```python
from build123d import *

# Parameters (mm, degrees)
F0_R     = 35.27027
F0_R_2   = 25.372409
F1_DEPTH = 50.8
F2_W     = 48.85688
F2_H     = 53.797463
F3_DEPTH = 25.4
F5_DEPTH = 5.08


with BuildPart() as f1:
    # F0 (on Top) → F1 (new body)
    with BuildSketch(Plane.XY):
        with Locations((0, 35.27027)):
            Circle(F0_R)
        with Locations((0, 35.27027)):
            Circle(F0_R_2, mode=Mode.SUBTRACT)
    extrude(amount=F1_DEPTH)

    # F2 (on Top) → F3 (join)
    with BuildSketch(Plane.XY):
        with Locations((0, -17.154805)):
            Rectangle(F2_W, F2_H)
    extrude(amount=F3_DEPTH)

    # F4 (on Right) → F5 (join, symmetric)
    with BuildSketch(Plane.YZ):
        Polygon((-27.996639, 25.663584), (4.117153, 25.389109), (4.117153, 41.857719), align=None)
    extrude(amount=F5_DEPTH, both=True)


solid = f1.part
```
Geometry check sheet. Reference: the model listing, model coordinates, mm. A direction names the side the tool comes from. Round coordinates to 2 decimals unless told otherwise and drop trailing zeros. Loops run counter-clockwise (first coordinate to the right, second up) from the corner with the lowest first, then second, coordinate; pieces in that order, holes last. Notation, with made-up numbers: (45, 52.25) -> (95, 52.25) arc R14 cw to (95, 76.25) -> close; hole circle Ø5 at (61, 11). An arc over 180 degrees is marked (long way). Use a Markdown table: item, result.
(1) Go/stop test with flat-tipped pins: P1, Ø12.5, axis at y = -28, z = 12.5, coming from the -X side; P2, Ø24.5, axis at x = -0.5, y = -17.5, coming from the +Z side; P3, Ø2, axis at y = 13, z = 22, coming from the +X side. Record where each tip stops, or that it passes through.
Calculated:
| item | result |
|---|---|
| P1 | x = -24.43 |
| P2 | z = 37.13 |
| P3 | x = 28.13 |
(2) Scan lines: probe 1 along Y at (x, z) = (0, 15); probe 2 along X at (y, z) = (-1, 12); probe 3 along Z at (x, y) = (-16, -33.5). Record each from-to range of solid material in increasing order.
Calculated:
| item | result |
|---|---|
| probe 1 | -44.05 to 9.9, 60.64 to 70.54 |
| probe 2 | -24.43 to 24.43 |
| probe 3 | 0 to 25.4 |
(3) Sectioned sample at A-A (y = 31). Enter the section's corners in (x, z), then the cut area to 3 significant figures.
Calculated:
| item | result |
|---|---|
| outline | (-35.01, 0) -> (-25.01, 0) -> (-25.01, 50.8) -> (-35.01, 50.8) -> close; (25.01, 0) -> (35.01, 0) -> (35.01, 50.8) -> (25.01, 50.8) -> close |
| area | 1,020 mm² |
(4) Sectioned sample at D-D (x = 22.5). Enter the section's corners in (y, z), then the cut area to 3 significant figures.
Calculated:
| item | result |
|---|---|
| outline | (-44.05, 0) -> (23.54, 0) -> (23.54, 50.8) -> (8.11, 50.8) -> (8.11, 25.4) -> (-44.05, 25.4) -> close; (47, 0) -> (62.43, 0) -> (62.43, 50.8) -> (47, 50.8) -> close |
| area | 2,890 mm² |
(5) Mould release check, pull along X, two halves, no side actions. Record for faces 6 (the flat face through (-5.08, -11, 30)), 7 (the flat face through (-24, 44, 50.8)), 8 (the cylindrical face through (-3.303, 60.427, 25.044)): released by +X, released by -X, zero draft, split by the parting line, or undercut.
Calculated:
| item | result |
|---|---|
| face 6 | released by -X |
| face 7 | zero draft |
| face 8 | undercut |
(6) Sectioned sample at C-C (z = 38.5). Enter the section's corners in (x, y).
Calculated:
| item | result |
|---|---|
| outline | (-5.08, -2.54) -> (5.08, -2.54) -> (5.08, 0.37) arc R35.27 ccw (long way) to (-5.08, 0.37) -> close; hole circle Ø50.74 at (0, 35.27) |
(7) Set-up check for faces 1 (the flat face through (0, 1, 0)), 2 (the flat face through (5.08, -11, 30)), 3 (the flat face through (0, -44.054, 13)), 4 (the flat face through (24.428, -18, 13)), 5 (the flat face through (-24.428, -18, 13)): record each of +Z, -Z, +X, -X, +Y, -Y from which the full face is reachable in a straight line by a thin tool's end or side.
Calculated:
| item | result |
|---|---|
| face 1 | -Z, +X, -X, +Y, -Y |
| face 2 | +Z, +X, -Y |
| face 3 | +Z, -Z, +X, -X, -Y |
| face 4 | +Z, -Z, +X, -Y |
| face 5 | +Z, -Z, -X, -Y |
